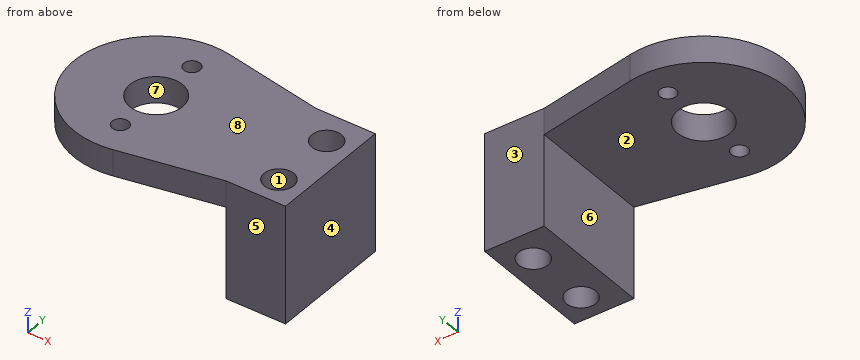
```python
from build123d import *

# Parameters (mm, degrees)
BOSS_EXTRUDE1_DEPTH = 4.000000656
SKETCH2_W           = 9.05
SKETCH2_H           = 18.8
BOSS_EXTRUDE2_DEPTH = 13.9
SKETCH3_R           = 4
SKETCH3_R_2         = 2.25
SKETCH3_R_3         = 1.25
CUT_EXTRUDE1_DEPTH  = 30


with BuildPart() as part:
    # Sketch1 → Boss-Extrude1 (new body)
    with BuildSketch(Plane(origin=(0, 0, 79.940542579), x_dir=(-1, 0, 0), z_dir=(0, 0, -1))):
        with BuildLine():
            Line((9.05, 0), (24.160371291, -2.879093513))
            ThreePointArc((24.160371291, -2.879093513), (39, 9.4), (24.160371291, 21.679093513))
            Line((24.160371291, 21.679093513), (9.05, 18.8))
            Line((9.05, 18.8), (0, 18.8))
            Line((0, 18.8), (0, 0))
            Line((0, 0), (9.05, 0))
        make_face()
    extrude(amount=-BOSS_EXTRUDE1_DEPTH)

    # Sketch2 → Boss-Extrude2 (add)
    with BuildSketch(Plane(origin=(0, 0, 79.940542579), x_dir=(-1, 0, 0), z_dir=(0, 0, -1))):
        with Locations((4.525, 9.4)):
            Rectangle(SKETCH2_W, SKETCH2_H)
    extrude(amount=BOSS_EXTRUDE2_DEPTH)

    # Sketch3 → Cut-Extrude1 (cut)
    with BuildSketch(Plane.XY.offset(83.940543234)):
        with Locations((-26.5, 9.4)):
            Circle(SKETCH3_R)
        with Locations((-3.95, 14.05)):
            Circle(SKETCH3_R_2)
        with Locations((-3.95, 4.05)):
            Circle(SKETCH3_R_2)
        with Locations((-26.5, 16.9)):
            Circle(SKETCH3_R_3)
        with Locations((-26.5, 1.9)):
            Circle(SKETCH3_R_3)
    extrude(amount=-CUT_EXTRUDE1_DEPTH, mode=Mode.SUBTRACT)


solid = part.part
```
For this review, take the finished solid that the model builds, in its own axes (mm). Face numbers are marked on the shaded views. A direction names the side the tool comes from. Round coordinates to 2 decimals unless told otherwise and drop trailing zeros. Write each loop counter-clockwise with the first axis right and the second up, starting at its lowest first coordinate (ties: lowest second). Pieces come first, ordered by that corner, then holes. Notation, with made-up numbers: (28, 25.25) -> (45, 25.25) arc R38 ccw to (45, 64.25) -> close; hole circle Ø9 at (27, 82). An arc over 180 degrees is marked (long way). One line per question, with ' | ' between items. Start each with the question number.
1) Add section A-A (x = -3.95). Write out the cut boundary in (y, z).
2) Mouldability with a two-part tool opening along X and no side actions: class the marked faces 6, 7 and 8 as +X half, -X half, draft (parallel to the pull), parting line (faces both ways), or undercut.
3) Add section B-B (z = 71.5). Write out the cut boundary in (x, y).
4) Machinability: for the marked faces 1, 2, 3, 4 and 5, which of the approach directions +Z, -Z, +X, -X, +Y, -Y give a long, thin tool a straight path to every point of the face, cutting with its end or side? Answer none if there is none.
5) Wall thickness on line 1 along Y through (x, z) = (-26.5, 80.8); line 2 along Y through (x, z) = (-3.95, 80); line 3 along X through (y, z) = (8, 68.5): over which ranges is each line inside the solid? List them lowest first.
6) For pin 1 Ø7.5 at (x, y) = (-22, 6.5) entering from -Z; pin 2 Ø4.5 at (x, z) = (-5, 71) entering from +Y; pin 3 Ø4 at (x, z) = (-15, 81) entering from -Y, all flat-tipped, find the tip position at first contact; note any pin that passes through.
7) Add section D-D (z = 81.25). Write out the cut boundary in (x, y), and give its area (3 significant figures).
8) Add section C-C (y = 9.4). Write out the cut boundary in (x, z), and give its area (3 significant figures).
Reported:
1) outline: (0, 66.04) -> (1.8, 66.04) -> (1.8, 83.94) -> (0, 83.94) -> close; (6.3, 66.04) -> (11.8, 66.04) -> (11.8, 83.94) -> (6.3, 83.94) -> close; (16.3, 66.04) -> (18.8, 66.04) -> (18.8, 83.94) -> (16.3, 83.94) -> close
2) face 6: -X half | face 7: undercut | face 8: draft
3) outline: (-9.05, 0) -> (0, 0) -> (0, 18.8) -> (-9.05, 18.8) -> close; hole circle Ø4.5 at (-3.95, 4.05); hole circle Ø4.5 at (-3.95, 14.05)
4) face 1: +Z, -Z | face 2: -Z, -X, +Y, -Y | face 3: +Z, -Z, +X, +Y | face 4: +Z, -Z, +X, +Y, -Y | face 5: +Z, -Z, +X, -Y
5) line 1: y = -3.1 to 0.65, 3.15 to 5.4, 13.4 to 15.65, 18.15 to 21.9 | line 2: y = 0 to 1.8, 6.3 to 11.8, 16.3 to 18.8 | line 3: x = -9.05 to 0
6) pin 1: stops at z = 79.94 | pin 2: stops at y = 18.8 | pin 3: stops at y = -1.51
7) outline: (-24.16, -2.88) -> (-9.05, 0) -> (0, 0) -> (0, 18.8) -> (-9.05, 18.8) -> (-24.16, 21.68) arc R12.5 ccw (long way) to start; hole circle Ø8 at (-26.5, 9.4); hole circle Ø2.5 at (-26.5, 1.9); hole circle Ø2.5 at (-26.5, 16.9); hole circle Ø4.5 at (-3.95, 4.05); hole circle Ø4.5 at (-3.95, 14.05) | area: 709 mm²
8) outline: (-39, 79.94) -> (-30.5, 79.94) -> (-30.5, 83.94) -> (-39, 83.94) -> close; (-22.5, 79.94) -> (-9.05, 79.94) -> (-9.05, 66.04) -> (0, 66.04) -> (0, 83.94) -> (-22.5, 83.94) -> close | area: 250 mm²
